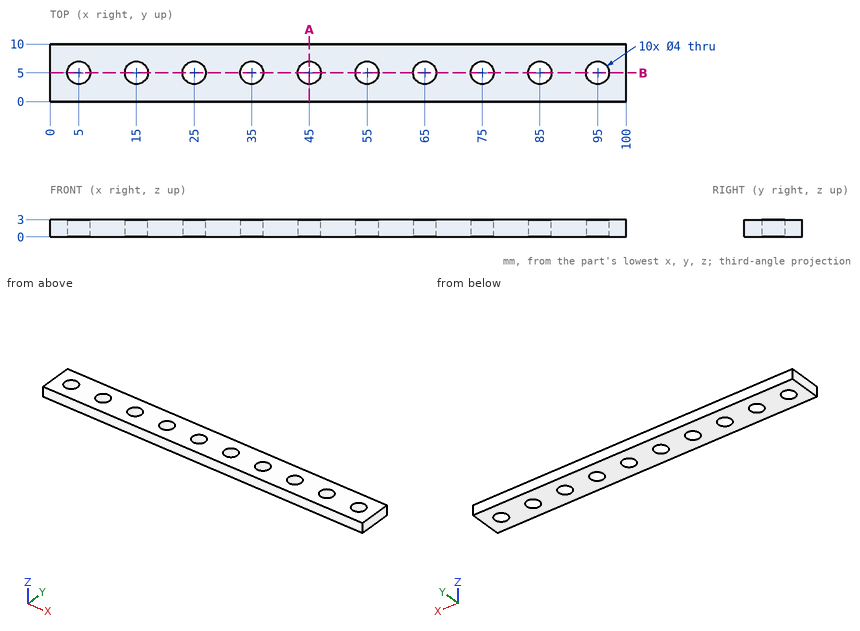
Print and shaded views of the part. All mm, measured from the part's lowest x, y and z. Round coordinates to 2 decimals unless told otherwise and drop trailing zeros. Write each loop counter-clockwise with the first axis right and the second up, starting at its lowest first coordinate (ties: lowest second). Pieces come first, ordered by that corner, then holes.
(1) Probe line 1 along Y through (x, z) = (85, 1.7); line 2 along Y through (x, z) = (95.5, 2.55). List the from-to ranges inside material, lowest first.
(2) Drop a flat-ended pin along its axis: P1, Ø3.5, axis at x = 35, y = 5, coming from the +Z side. Give the stop position or say it passes through.
(3) Slice it at B-B, the plane y = 5. Count the separate pieces of the cut face and the enclosed holes in it, and give its area (3 significant figures).
(4) Slice it at A-A, the plane x = 45. Write the cut outline in (y, z).
From the geometry:
1. line 1: y = 0 to 3, 7 to 10
1. line 2: y = 0 to 3.06, 6.94 to 10
2. P1: passes through
3. separate pieces: 11
3. enclosed holes: 0
3. area: 180 mm2
4. outline: (0, 0) - (3, 0) - (3, 3) - (0, 3) - close; (7, 0) - (10, 0) - (10, 3) - (7, 3) - close
